Input: part model. Units: mm. Frame: model coordinates. Face numbers are marked on the shaded views. A direction names the side the tool comes from. Coordinates: 2 decimals unless noted, no trailing zeros. Write each loop counter-clockwise with the first axis right and the second up, starting at its lowest first coordinate (ties: lowest second). Pieces come first, ordered by that corner, then holes.
1) Section query D-D (x = 36.5). Output: boundary loops of the cut face in (y, z) (3 decimals).
2) Section query A-A (x = 48.26). Output: boundary loops of the cut face in (y, z) (3 decimals).
3) Set-up query: the marked faces 1, 2 and 3. Return all of +Z, -Z, +X, -X, +Y, -Y with unobstructed straight access to the full face (end or side cutting, diameter ignored); none if empty.
4) Section query B-B (y = 0). Output: boundary loops of the cut face in (x, z) (3 decimals), then the cut area to 3 significant figures.
5) Section query C-C (z = 0). Output: boundary loops of the cut face in (x, y) (3 decimals), then the cut area to 3 significant figures.
6) Pin query (flat end, axial travel): pin 1 Ø1 at (x, y) = (15, 2.5) entering from +Z; pin 2 Ø1 at (x, y) = (20.5, 2) entering from +Z; pin 3 Ø1 at (x, z) = (22.5, -2) entering from +Y. Return the tip coordinate at first contact, or that it passes through.
7) Line query: L1, parallel to Y at x = 48.26, z = -0.9; L2, parallel to Y at x = 48.26, z = 1; L3, parallel to X at y = 1.5, z = -0.25. Output: solid intervals per line, ascending.
from build123d import *

# Parameters (mm, degrees)
F0_R     = 2.54
F1_DEPTH = 50.8
F3_DEPTH = 12.7
F4_W     = 5.3957496343
F4_H     = 1.27
F5_DEPTH = 5.588
F6_R     = 1.27
F7_DEPTH = 25.4
F9_START = -12.7
F8_R     = 3.175
F9_DEPTH = 2.54


with BuildPart() as f1:
    # F0 (on Right) → F1 (new body)
    with BuildSketch(Plane.YZ):
        Circle(F0_R)
    extrude(amount=F1_DEPTH)

    # F2 (on face) → F3 (cut)
    with BuildSketch(Plane.YZ.offset(50.8)):
        with BuildLine():
            Line((1.7070901198, -3.1991907798), (1.7070901198, -1.8808092202))
            ThreePointArc((1.7070901198, -1.8808092202), (0, -2.54), (-1.7070901198, -1.8808092202))
            Line((-1.7070901198, -1.8808092202), (-1.7070901198, -3.1991907798))
            Line((-1.7070901198, -3.1991907798), (1.7070901198, -3.1991907798))
        make_face()
        with BuildLine():
            ThreePointArc((-1.7070901198, -1.8808092202), (0, -2.54), (1.7070901198, -1.8808092202))
            Line((1.7070901198, -1.8808092202), (-1.7070901198, -1.8808092202))
        make_face()
        with BuildLine():
            Line((-1.7070901198, 1.8808092202), (1.7070901198, 1.8808092202))
            ThreePointArc((1.7070901198, 1.8808092202), (0, 2.54), (-1.7070901198, 1.8808092202))
        make_face()
        with BuildLine():
            ThreePointArc((-1.7070901198, 1.8808092202), (0, 2.54), (1.7070901198, 1.8808092202))
            Line((1.7070901198, 1.8808092202), (1.7070901198, 3.1991907798))
            Line((1.7070901198, 3.1991907798), (-1.7070901198, 3.1991907798))
            Line((-1.7070901198, 3.1991907798), (-1.7070901198, 1.8808092202))
        make_face()
    extrude(amount=-F3_DEPTH, mode=Mode.SUBTRACT)

    # F4 (on face) → F5 (cut)
    with BuildSketch(Plane.YZ.offset(50.8)):
        Rectangle(F4_W, F4_H)
    extrude(amount=-F5_DEPTH, mode=Mode.SUBTRACT)

    # F6 (on face) → F7 (cut)
    with BuildSketch(Plane.XY.offset(1.8808092202)):
        with Locations((48.26, 0)):
            Circle(F6_R)
    extrude(amount=-F7_DEPTH, mode=Mode.SUBTRACT)

    # F8 (on face) → F9 (join)
    with BuildSketch(Plane.YZ.offset(50.8).offset(F9_START)):
        Circle(F8_R)
        with BuildLine():
            Line((2.4593444248, 0.635), (-2.4593444248, 0.635))
            ThreePointArc((-2.4593444248, 0.635), (-2.1743514797, 1.3129339827), (-1.7070901198, 1.8808092202))
            Line((-1.7070901198, 1.8808092202), (1.7070901198, 1.8808092202))
            ThreePointArc((1.7070901198, 1.8808092202), (2.1743514797, 1.3129339827), (2.4593444248, 0.635))
        make_face(mode=Mode.SUBTRACT)
    extrude(amount=-F9_DEPTH)


solid = f1.part
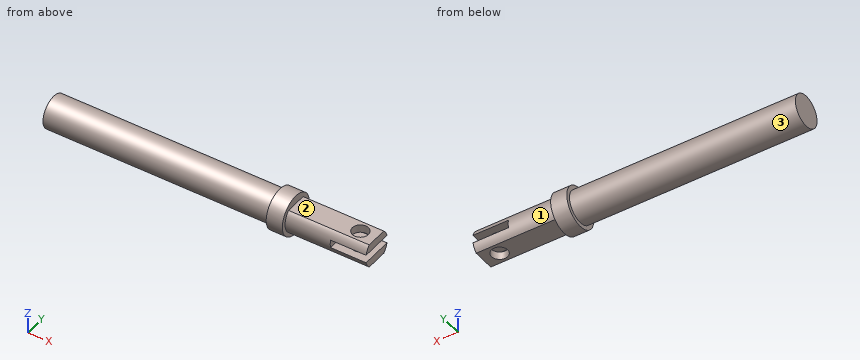
Answer:
1. outline: circle Ø6.35 at (0, 0)
2. outline: (-2.459, -0.635) arc R2.54 ccw to (-1.707, -1.881) - (-1.27, -1.881) - (-1.27, -0.635) - close; (-2.459, 0.635) - (-1.27, 0.635) - (-1.27, 1.881) - (-1.707, 1.881) arc R2.54 ccw to start; (1.27, -1.881) - (1.707, -1.881) arc R2.54 ccw to (2.459, -0.635) - (1.27, -0.635) - close; (1.27, 0.635) - (2.459, 0.635) arc R2.54 ccw to (1.707, 1.881) - (1.27, 1.881) - close
3. face 1: +X, +Y
3. face 2: +Z, +X, +Y, -Y
3. face 3: -X
4. outline: (0, -2.54) - (35.56, -2.54) - (35.56, -3.175) - (38.1, -3.175) - (38.1, -1.881) - (46.99, -1.881) - (46.99, -0.635) - (45.212, -0.635) - (45.212, 0.635) - (46.99, 0.635) - (46.99, 1.881) - (38.1, 1.881) - (38.1, 3.175) - (35.56, 3.175) - (35.56, 2.54) - (0, 2.54) - close; (49.53, -1.881) - (50.8, -1.881) - (50.8, -0.635) - (49.53, -0.635) - close; (49.53, 0.635) - (50.8, 0.635) - (50.8, 1.881) - (49.53, 1.881) - close
4. area: 231 mm2
5. outline: (0, -2.54) - (35.56, -2.54) - (35.56, -3.175) - (38.1, -3.175) - (38.1, -2.54) - (45.212, -2.54) - (45.212, 2.54) - (38.1, 2.54) - (38.1, 3.175) - (35.56, 3.175) - (35.56, 2.54) - (0, 2.54) - close
5. area: 233 mm2
6. pin 1: stops at z = 1.57
6. pin 2: stops at z = 2.05
6. pin 3: stops at y = 2.05
7. L1: y = -2.38 to -1.27, 1.27 to 2.38
7. L2: y = -2.33 to -1.27, 1.27 to 2.33
7. L3: x = 0 to 45.21
